from build123d import *

# Parameters (mm, degrees)
BOSS_EXTRUDE1_DEPTH = 20.5
SKETCH2_R           = 9.225
BOSS_EXTRUDE2_DEPTH = 0.75
SKETCH3_R           = 9.75
BOSS_EXTRUDE3_DEPTH = 1.85
SKETCH4_R           = 6.6
BOSS_EXTRUDE4_DEPTH = 10
SKETCH5_R           = 3.8
CUT_EXTRUDE1_DEPTH  = 37.207814534
SKETCH6_R           = 5.5
CUT_EXTRUDE2_DEPTH  = 16.5


with BuildPart() as part:
    # Sketch1 → Boss-Extrude1 (new body)
    with BuildSketch(Plane(origin=(0, 0, 0), x_dir=(1, 0, 0), z_dir=(0, 1, 0))):
        Polygon((-9.5, 5.484827557), (-9.5, -5.484827557), (0, -10.969655115), (9.5, -5.484827557), (9.5, 5.484827557), (0, 10.969655115), align=None)
    extrude(amount=BOSS_EXTRUDE1_DEPTH)

    # Sketch2 → Boss-Extrude2 (add)
    with BuildSketch(Plane(origin=(0, 20.5, 0), x_dir=(1, 0, 0), z_dir=(0, 1, 0))):
        with Locations(Location((0, 0, 0), (0, 0, 270))):
            Circle(SKETCH2_R)
    extrude(amount=BOSS_EXTRUDE2_DEPTH)

    # Sketch3 → Boss-Extrude3 (add)
    with BuildSketch(Plane(origin=(0, 21.25, 0), x_dir=(1, 0, 0), z_dir=(0, 1, 0))):
        with Locations(Location((0, 0, 0), (0, 0, 270))):
            Circle(SKETCH3_R)
    extrude(amount=BOSS_EXTRUDE3_DEPTH)

    # Sketch4 → Boss-Extrude4 (add)
    with BuildSketch(Plane(origin=(0, 23.1, 0), x_dir=(1, 0, 0), z_dir=(0, 1, 0))):
        with Locations(Location((0, 0, 0), (0, 0, 270))):
            Circle(SKETCH4_R)
    extrude(amount=BOSS_EXTRUDE4_DEPTH)

    # Sketch5 → Cut-Extrude1 (cut, through all)
    with BuildSketch(Plane(origin=(0, 33.1, 0), x_dir=(1, 0, 0), z_dir=(0, 1, 0))):
        with Locations(Location((0, 0, 0), (0, 0, 270))):
            Circle(SKETCH5_R)
    extrude(amount=-CUT_EXTRUDE1_DEPTH, mode=Mode.SUBTRACT)

    # Sketch6 → Cut-Extrude2 (cut)
    with BuildSketch(Plane.XZ):
        with Locations(Location((0, 0, 0), (0, 0, 270))):
            Circle(SKETCH6_R)
    extrude(amount=-CUT_EXTRUDE2_DEPTH, mode=Mode.SUBTRACT)

    # Sketch7 → Revolve1 (revolve)
    with BuildSketch(Plane.XY, mode=Mode.PRIVATE) as revolve1_sk:
        with BuildLine():
            Line((-6.6, 23.6), (-6.6, 23.1))
            Line((-6.6, 23.1), (-7.1, 23.1))
            ThreePointArc((-7.1, 23.1), (-6.953553391, 23.453553391), (-6.6, 23.6))
        make_face()
    revolve(revolve1_sk.sketch.rotate(Axis((0, 0, 0), (0, 1, 0)), 270), axis=Axis((0, 0, 0), (0, 1, 0)))


solid = part.part
The model under review builds one solid part; all positions refer to its coordinate system, in mm. A direction names the side the tool comes from. Round coordinates to 2 decimals unless told otherwise and drop trailing zeros. Loops run counter-clockwise (first coordinate to the right, second up) from the corner with the lowest first, then second, coordinate; pieces in that order, holes last. Notation, with made-up numbers: (42, 72.5) -> (65, 72.5) arc R5 ccw to (65, 78.5) -> close; hole circle Ø8 at (19, -21.75). An arc over 180 degrees is marked (long way). Write item = value, one per line. Start each with the question number.
Item 1: Take a section at C-C on z = 8. Give the boundary of the cut face in (x, y).
Item 2: Insertion check: pin 1 (5.5 mm diameter, centred on y = 9.5, z = 1, fed in from -X); pin 2 (5 mm diameter, centred on y = 13.5, z = 8.5, fed in from +X); pin 3 (12 mm diameter, centred on y = 12, z = -1, fed in from +X); pin 4 (7 mm diameter, centred on x = 0, z = 0, fed in from -Y). Each pin has a flat end and moves straight along its axis. Give the tip position at first contact, or say it passes through.
Item 3: Mouldability with a two-part tool opening along X and no side actions: class faces 1 (the cylindrical face through (9.667, 22.162, -1.269)), 2 (the flat face through (-4, 0, 5)), 3 (the flat face through (9.5, 10, 0)), 4 (the flat face through (1, 16.5, -4)) as released by +X, released by -X, zero draft, split by the parting line, or undercut.
Item 4: Take a section at D-D on x = -8. Give the boundary of the cut face in (y, z), plus the area to 3 significant figures.
Item 5: Take a section at A-A on z = 0. Give the boundary of the cut face in (x, y) (3 decimals).
Item 6: For faces 5 (the cylindrical face through (-5.37, 8.13, 1.19)), 6 (the flat face through (-4.8, 10.1, 8.2)), 7 (the flat face through (-9.5, 10, 0)), 8 (the cylindrical face through (2.77, 20.87, 8.8)), list the 3-axis set-ups (+Z, -Z, +X, -X, +Y, -Y) from which the entire face can be reached by the end or side of a thin tool; tool diameter is ignored.
Item 7: To check wall thickness, follow L1, parallel to X at y = 8, z = 0; L2, parallel to X at y = 29.75, z = 0; L3, parallel to Z at x = 3, y = 9.5. State the ranges of each line that lie inside material, in increasing order.
Item 8: Take a section at B-B on y = 15. Give the boundary of the cut face in (x, z).
Result:
q1.outline = (-5.57, 21.25) -> (-4.59, 21.25) -> (-4.59, 20.5) -> (-5.14, 20.5) -> (-5.14, 0) -> (5.14, 0) -> (5.14, 20.5) -> (4.59, 20.5) -> (4.59, 21.25) -> (5.57, 21.25) -> (5.57, 23.1) -> (-5.57, 23.1) -> close
q2.pin_1 = -9.5
q2.pin_2 = 8.61
q2.pin_3 = 9.5
q2.pin_4 = through
q3.face_1 = split by the parting line
q3.face_2 = zero draft
q3.face_3 = released by +X
q3.face_4 = undercut
q4.outline = (0, -6.35) -> (20.5, -6.35) -> (20.5, -4.59) -> (21.25, -4.59) -> (21.25, -5.57) -> (23.1, -5.57) -> (23.1, 5.57) -> (21.25, 5.57) -> (21.25, 4.59) -> (20.5, 4.59) -> (20.5, 6.35) -> (0, 6.35) -> close
q4.area = 288 mm²
q5.outline = (-9.75, 21.25) -> (-9.225, 21.25) -> (-9.225, 20.5) -> (-9.5, 20.5) -> (-9.5, 0) -> (-5.5, 0) -> (-5.5, 16.5) -> (-3.8, 16.5) -> (-3.8, 33.1) -> (-6.6, 33.1) -> (-6.6, 23.6) arc R0.5 ccw to (-7.1, 23.1) -> (-9.75, 23.1) -> close; (3.8, 16.5) -> (5.5, 16.5) -> (5.5, 0) -> (9.5, 0) -> (9.5, 20.5) -> (9.225, 20.5) -> (9.225, 21.25) -> (9.75, 21.25) -> (9.75, 23.1) -> (7.1, 23.1) arc R0.5 ccw to (6.6, 23.6) -> (6.6, 33.1) -> (3.8, 33.1) -> close
q6.face_5 = -Y
q6.face_6 = +Z, -X, -Y
q6.face_7 = +Z, -Z, -X, -Y
q6.face_8 = none
q7.L1 = -9.5 to -5.5, 5.5 to 9.5
q7.L2 = -6.6 to -3.8, 3.8 to 6.6
q7.L3 = -9.24 to -4.61, 4.61 to 9.24
q8.outline = (-9.5, -5.48) -> (0, -10.97) -> (9.5, -5.48) -> (9.5, 5.48) -> (0, 10.97) -> (-9.5, 5.48) -> close; hole circle Ø11 at (0, 0)
